from build123d import *

# Parameters (mm, degrees)
F0_R     = 30
F0_R_2   = 1.5
F0_R_3   = 4
F1_DEPTH = 12
F2_SIZE  = 1
F3_R     = 10
F4_DEPTH = 2


with BuildPart() as f1:
    # F0 (on Top) → F1 (new body)
    with BuildSketch(Plane.XY):
        Circle(F0_R)
        with Locations((-10.606602, -10.606602)):
            Circle(F0_R_2, mode=Mode.SUBTRACT)
        with Locations((10.606602, -10.606602)):
            Circle(F0_R_2, mode=Mode.SUBTRACT)
        with Locations((-10.606602, 10.606602)):
            Circle(F0_R_2, mode=Mode.SUBTRACT)
        Circle(F0_R_3, mode=Mode.SUBTRACT)
        with Locations((10.606602, 10.606602)):
            Circle(F0_R_2, mode=Mode.SUBTRACT)
    extrude(amount=F1_DEPTH)

    # F2
    f2_edges = [f1.edges().sort_by_distance(p)[0] for p in [
        (-30, 0, 0),
    ]]
    chamfer(f2_edges, length=F2_SIZE)

    # F3 (on face) → F4 (cut)
    with BuildSketch(Plane(origin=(0, 0, 0), x_dir=(1, 0, 0), z_dir=(0, 0, -1))):
        Circle(F3_R)
    extrude(amount=-F4_DEPTH, mode=Mode.SUBTRACT)


solid = f1.part
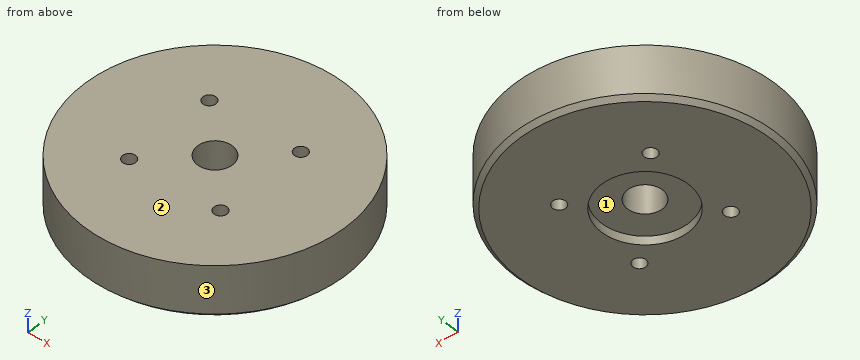
Here's how the part is built. I have some questions about the finished solid (model axes, mm). Face numbers are marked on the shaded views. Give positions to 0.01 mm unless a question says otherwise; leave off trailing zeros. Loops run counter-clockwise (first coordinate to the right, second up) from the corner with the lowest first, then second, coordinate; pieces in that order, holes last. Notation, with made-up numbers: (11, 6.5) -> (66, 6.5) arc R29 ccw to (66, 37.5) -> close; hole circle Ø6 at (48, 54.5). An arc over 180 degrees is marked (long way). One line per item, written item: value.
Q1. If I drill on line 1 along Y through (x, z) = (0, 4.75); line 2 along Y through (x, z) = (11, 6.5); line 3 along X through (y, z) = (11.5, 7.75), over which ranges is the centre line in solid material (lowest first)?
Answers follow:
line 1: -30 to -4, 4 to 30
line 2: -27.91 to -12.05, -9.16 to 9.16, 12.05 to 27.91
line 3: -27.71 to -11.81, -9.4 to 9.4, 11.81 to 27.71
Q2. Suppose I cut it at A-A on y = 0. Please give me the cut outline in (x, z), then the cut area to 3 significant figures.
Answers follow:
outline: (-30, 1) -> (-29, 0) -> (-10, 0) -> (-10, 2) -> (-4, 2) -> (-4, 12) -> (-30, 12) -> close; (4, 2) -> (10, 2) -> (10, 0) -> (29, 0) -> (30, 1) -> (30, 12) -> (4, 12) -> close
area: 599 mm^2
Q3. I'm going to push flat-ended pins straight in: pin 1 Ø1.5 at (y, z) = (2, 8) entering from -X; pin 2 Ø6 at (y, z) = (-22, 4) entering from -X; pin 3 Ø9 at (x, y) = (0, 0) entering from -Z. Where does each tip first touch, or does it pass through?
Answers follow:
pin 1: x = -29.97
pin 2: x = -23.22
pin 3: z = 2
Q4. We'd pull the mould along Y, two halves only. Please class the marked faces 1, 2 and 3: pulls with the +Y half, pulls with the -Y half, needs draft (parallel to the pull), parting line crosses it, or undercut.
Answers follow:
face 1: undercut
face 2: needs draft
face 3: parting line crosses it
Q5. Suppose I cut it at C-C on z = 11.25. Please give me the cut outline in (x, y).
Answers follow:
outline: circle Ø60 at (0, 0); hole circle Ø3 at (-10.61, -10.61); hole circle Ø3 at (-10.61, 10.61); hole circle Ø8 at (0, 0); hole circle Ø3 at (10.61, -10.61); hole circle Ø3 at (10.61, 10.61)
